Here's how the part is built. I have some questions about the finished solid (model axes, mm). A direction names the side the tool comes from. Round coordinates to 2 decimals unless told otherwise and drop trailing zeros. Order: outer loops, then holes, each group sorted by start corner. A loop starts at its lowest first (then second) coordinate and runs counter-clockwise, first axis right, second up. Notation, with made-up numbers: (72, 53.5) -> (94, 53.5) arc R13 cw to (94, 71.5) -> close; hole circle Ø4 at (26.5, -6). An arc over 180 degrees is marked (long way). One line per item, written item: value.
```python
from build123d import *

# Parameters (mm, degrees)
SKETCH1_R           = 2
SKETCH1_W           = 22.75
SKETCH1_H           = 11.5
BOSS_EXTRUDE1_DEPTH = 3.175
FILLET1_R           = 3.175


with BuildPart() as part:
    # Sketch1 → Boss-Extrude1 (new body)
    with BuildSketch(Plane(origin=(0, 0, 0), x_dir=(1, 0, 0), z_dir=(0, 1, 0))):
        Polygon((0, 0), (70, 0), (70, 22.5425), (63.575, 22.5425), (63.575, 25.7175), (57.225, 25.7175), (57.225, 22.5425), (50.875, 22.5425), (50.875, 25.7175), (44.525, 25.7175), (44.525, 22.5425), (38.175, 22.5425), (38.175, 25.7175), (31.825, 25.7175), (31.825, 22.5425), (25.475, 22.5425), (25.475, 25.7175), (19.125, 25.7175), (19.125, 22.5425), (12.775, 22.5425), (12.775, 25.7175), (6.425, 25.7175), (6.425, 22.5425), (0, 22.5425), align=None)
        with Locations(Location((26, 7.3375, 0), (0, 0, 270))):
            Circle(SKETCH1_R, mode=Mode.SUBTRACT)
        with Locations(Location((55.75, 7.3375, 0), (0, 0, 90))):
            Circle(SKETCH1_R, mode=Mode.SUBTRACT)
        with Locations((40.875, 7.3375)):
            Rectangle(SKETCH1_W, SKETCH1_H, mode=Mode.SUBTRACT)
    extrude(amount=BOSS_EXTRUDE1_DEPTH)

    # Fillet1
    fillet1_edges = [part.edges().sort_by_distance(p)[0] for p in [
        (70, 1.5875, 0),
        (0, 1.5875, 0),
    ]]
    fillet(fillet1_edges, radius=FILLET1_R)


solid = part.part
```
Q1. I want a section at C-C on y = 0.9. Give the number of separate pieces and of enclosed holes in the cut face, then the cut area to 3 significant figures.
Answers:
separate pieces: 1
enclosed holes: 3
area: 1,390 mm2
Q2. For P1, Ø1.6, axis at x = 66, y = 1.5, coming from the -Z side; P2, Ø1.6, axis at y = 1.5, z = -24, coming from the -X side (3 decimals); P3, Ø1, axis at y = 1, z = -24, coming from the +X side (3 decimals), each with a flat end and sliding along its axis, tell me the tip position at first contact or that it passes through.
Answers:
P1: z = -22.54
P2: x = 6.425
P3: x = 63.575
Q3. If we mould it in two halves opening along X, with no side actions, what happens to faces 1 (the face through (22, 2, -25.718)), 2 (the face through (16, 2, -22.542)), 3 (the face through (69.05, 1.61, -0.91)), 4 (the face through (25.475, 2, -24))? For each: pulls with the +X half, pulls with the -X half, needs draft (parallel to the pull), parting line crosses it, or undercut.
Answers:
face 1: needs draft
face 2: undercut
face 3: pulls with the +X half
face 4: undercut
Q4. I want a section at B-B on z = -4.5. Write out the boundary of the cut face in (x, y) (3 decimals), then the cut area to 3 significant figures.
Answers:
outline: (0, 0) -> (29.5, 0) -> (29.5, 3.175) -> (0, 3.175) -> close; (52.25, 0) -> (70, 0) -> (70, 3.175) -> (52.25, 3.175) -> close
area: 150 mm2
Q5. I want a section at A-A on x = 55.75. Write out the boundary of the cut face in (y, z) (1 decimal).
Answers:
outline: (0, -22.5) -> (3.2, -22.5) -> (3.2, -9.3) -> (0, -9.3) -> close; (0, -5.3) -> (3.2, -5.3) -> (3.2, 0) -> (0, 0) -> close
Q6. Which directions (+Z, -Z, +X, -X, +Y, -Y) give clear straight access to the entire face, cutting with the end or side of a thin tool? Please do faces 5 (the face through (63.575, 2, -24)), 6 (the face through (41, 2, -1.588)), 7 (the face through (29, 2, -22.542)).
Answers:
face 5: -Z, +X, +Y, -Y
face 6: +Y, -Y
face 7: -Z, +Y, -Y
Q7. I need wall thicknesses on line 1 along X through (y, z) = (0.6, -22.75) (3 decimals); line 2 along Z through (x, y) = (55.75, 2.1); line 3 along Z through (x, y) = (35, 1.2). Which ranges of each line are inside material? Lowest first, please.
Answers:
line 1: 6.425 to 12.775, 19.125 to 25.475, 31.825 to 38.175, 44.525 to 50.875, 57.225 to 63.575
line 2: -22.54 to -9.34, -5.34 to 0
line 3: -25.72 to -13.09, -1.59 to 0
